from build123d import *

# Parameters (mm, degrees)
SKETCH1_W           = 29.21
SKETCH1_H           = 29.21
SKETCH1_W_2         = 26.035
SKETCH1_H_2         = 26.035
BOSS_EXTRUDE1_DEPTH = 101.6
SKETCH2_R           = 8
CUT_EXTRUDE1_DEPTH  = 50.8
BOSS_EXTRUDE2_DEPTH = 26.035
SKETCH6_R           = 10.16
SKETCH6_R_2         = 8
BOSS_EXTRUDE3_DEPTH = 5.08
FILLET1_R           = 2.54
SKETCH7_R           = 2.25
CUT_EXTRUDE2_DEPTH  = 46.736
SKETCH8_W           = 26.035
SKETCH8_H           = 26.035
SKETCH8_W_2         = 22.86
SKETCH8_H_2         = 22.86
BOSS_EXTRUDE4_DEPTH = 1


with BuildPart() as part:
    # Sketch1 → Boss-Extrude1 (new body)
    with BuildSketch(Plane(origin=(0, 0, 0), x_dir=(1, 0, 0), z_dir=(0, 1, 0))):
        Rectangle(SKETCH1_W, SKETCH1_H)
        Rectangle(SKETCH1_W_2, SKETCH1_H_2, mode=Mode.SUBTRACT)
    extrude(amount=BOSS_EXTRUDE1_DEPTH)

    # Sketch2 → Cut-Extrude1 (cut)
    with BuildSketch(Plane.XY.offset(14.605)):
        with BuildLine():
            Line((-14.605, 101.6), (-14.605, 38.1))
            ThreePointArc((-14.605, 38.1), (0, 52.705), (14.605, 38.1))
            Line((14.605, 38.1), (14.605, 101.6))
            Line((14.605, 101.6), (-14.605, 101.6))
        make_face()
        with Locations((0, 38.1)):
            Circle(SKETCH2_R)
    extrude(amount=-CUT_EXTRUDE1_DEPTH, mode=Mode.SUBTRACT)

    # Sketch5 → Boss-Extrude2 (add)
    with BuildSketch(Plane.XY.offset(-13.0175)):
        with BuildLine():
            Line((-13.0175, 44.721987523), (-13.0175, 38.1))
            ThreePointArc((-13.0175, 38.1), (0, 51.1175), (13.0175, 38.1))
            Line((13.0175, 38.1), (13.0175, 44.721987523))
            ThreePointArc((13.0175, 44.721987523), (0, 52.705), (-13.0175, 44.721987523))
        make_face()
    extrude(amount=BOSS_EXTRUDE2_DEPTH)

    # Sketch6 → Boss-Extrude3 (add)
    with BuildSketch(Plane(origin=(0, 0, 13.0175), x_dir=(-1, 0, 0), z_dir=(0, 0, -1))):
        with Locations((0, 38.1)):
            Circle(SKETCH6_R)
        with Locations(Location((0, 38.1, 0), (0, 0, 180))):
            Circle(SKETCH6_R_2, mode=Mode.SUBTRACT)
    extrude(amount=BOSS_EXTRUDE3_DEPTH)

    # Fillet1
    fillet1_edges = [part.edges().sort_by_distance(p)[0] for p in [
        (10.16, 38.1, 13.0175),
    ]]
    fillet(fillet1_edges, radius=FILLET1_R)

    # Mirror7: part across plane


with BuildPart() as part_1:
    add(part.part)
    add(part.part.mirror(Plane.XY))

    # Sketch7 → Cut-Extrude2 (cut)
    with BuildSketch(Plane(origin=(0, 0, -14.605), x_dir=(-1, 0, 0), z_dir=(0, 0, -1))):
        with Locations((-8.255, 8.7)):
            Circle(SKETCH7_R)
        with Locations((8.255, 4)):
            Circle(SKETCH7_R)
    extrude(amount=-CUT_EXTRUDE2_DEPTH, mode=Mode.SUBTRACT)

    # Sketch8 → Boss-Extrude4 (add)
    with BuildSketch(Plane(origin=(0, 25.4, 0), x_dir=(-1, 0, 0), z_dir=(0, -1, 0))):
        Rectangle(SKETCH8_W, SKETCH8_H)
        Rectangle(SKETCH8_W_2, SKETCH8_H_2, mode=Mode.SUBTRACT)
    extrude(amount=-BOSS_EXTRUDE4_DEPTH)


solid = part_1.part
Read the model definition and answer for the solid it produces. Units are mm, in the model's axes. A direction names the side the tool comes from. Coordinates: 2 decimals unless noted, no trailing zeros. Loops run counter-clockwise (first coordinate to the right, second up) from the corner with the lowest first, then second, coordinate; pieces in that order, holes last. Notation, with made-up numbers: (-2, -35) -> (28, -35) arc R32 ccw to (28, -4) -> close; hole circle Ø3 at (19.5, -34). An arc over 180 degrees is marked (long way). Write item = value, one per line. Start each with the question number.
1) The part is cut by section C-C, the plane x = 0. State how many separate pieces and enclosed holes the cut face has, plus the area to 3 significant figures.
2) The part is cut by section B-B, the plane y = 8.7. Determine the outline of the cut face in (x, z) (1 decimal), plus the area to 3 significant figures.
3) The part is cut by section D-D, the plane y = 21. Determine the outline of the cut face in (x, z) (1 decimal).
4) For faces 1 (the face through (0, 29.9, 7.938)), 2 (the face through (12, 26.4, 0)), 3 (the face through (-1.041, 30.168, 11.318)), determine the directions among +Z, -Z, +X, -X, +Y, -Y from which every point of the face is accessible in a straight line to the end or side of a thin tool.
5) Find the intervals of material crossed by L1, parallel to X at y = 34, z = -1.75 (1 decimal); L2, parallel to Y at x = 0.25, z = -8.5, in increasing order. Write a range as from..to.
6) Given P1, Ø4, axis at x = -8.255, y = 4, coming from the -Z side; P2, Ø5, axis at y = 42, z = 8, coming from the -X side; P3, Ø6, axis at x = 7, z = -0.5, coming from the -Y side; P4, Ø1, axis at x = 8.5, z = -0.5, coming from the +Y side, each flat-ended and moving along its own axis, determine where each tip first touches the part or whether it passes through.
7) The part is cut by section A-A, the plane z = -9.5. Determine the outline of the cut face in (x, y) (1 decimal).
8) The mould has two halves that part along X. Classify faces 4 (the face through (0, 13, -13.018)), 5 (the face through (-14.605, 19, 0)), 6 (the face through (0, 26, -14.605)): pulls with the +X half, pulls with the -X half, needs draft (parallel to the pull), parting line crosses it, or undercut.
Result:
q1.separate_pieces = 3
q1.enclosed_holes = 0
q1.area = 210 mm²
q2.outline = (-14.6, -14.6) -> (6, -14.6) -> (6, -13) -> (-13, -13) -> (-13, 13) -> (6, 13) -> (6, 14.6) -> (-14.6, 14.6) -> close; (10.5, -14.6) -> (14.6, -14.6) -> (14.6, 14.6) -> (10.5, 14.6) -> (10.5, 13) -> (13, 13) -> (13, -13) -> (10.5, -13) -> close
q2.area = 161 mm²
q3.outline = (-14.6, -14.6) -> (14.6, -14.6) -> (14.6, 14.6) -> (-14.6, 14.6) -> close; hole (-13, -13) -> (13, -13) -> (13, 13) -> (-13, 13) -> close
q4.face_1 = -Y
q4.face_2 = none
q4.face_3 = +Z, -Z
q5.L1 = -14.6..-13, 13..14.6
q5.L2 = 27.94..30.1, 46.1..48.26, 51.12..52.7
q6.P1 = through
q6.P2 = -14.54
q6.P3 = 46.43
q6.P4 = 50.32
q7.outline = (-14.6, 0) -> (-13, 0) -> (-13, 25.4) -> (-11.4, 25.4) -> (-11.4, 26.4) -> (-13, 26.4) -> (-13, 38.1) arc R13 cw to (13, 38.1) -> (13, 26.4) -> (11.4, 26.4) -> (11.4, 25.4) -> (13, 25.4) -> (13, 0) -> (14.6, 0) -> (14.6, 38.1) arc R14.6 ccw to (-14.6, 38.1) -> close; circle Ø20.3 at (0, 38.1); hole circle Ø16 at (0, 38.1)
q8.face_4 = undercut
q8.face_5 = pulls with the -X half
q8.face_6 = needs draft
